Could you check a few things on this model? Use its own coordinates, in mm. Face numbers are marked on the shaded views. Give positions to 0.01 mm unless a question says otherwise; leave off trailing zeros. Loops run counter-clockwise (first coordinate to the right, second up) from the corner with the lowest first, then second, coordinate; pieces in that order, holes last.
1. Imagine slicing it at A-A (z = 0). List the corners of the cut face in (x, y) for me, plus the area to 4 significant figures.
2. Imagine slicing it at B-B (y = 1.5). List the corners of the cut face in (x, z) for me.
3. For P1, Ø2, axis at x = -12.5, z = 0, coming from the +Y side; P2, Ø4, axis at y = 7, z = 10.5, coming from the -X side; P3, Ø5, axis at y = 2, z = -7, coming from the +X side; P4, Ø3, axis at x = 0, z = 12.5, coming from the -Y side, each with a flat end and sliding along its axis, tell me the tip position at first contact or that it passes through.
4. Thinking about a two-plate mould opening in Z: for the marked faces 1, 2 and 3, which applies, +Z half, -Z half, draft (parallel to the pull), parting line (faces both ways), or undercut?
5. Imagine slicing it at D-D (z = -12.5). List the corners of the cut face in (x, y) for me.
6. I need wall thicknesses on line 1 along X through (y, z) = (6.5, 0); line 2 along X through (y, z) = (3.75, 1); line 3 along X through (y, z) = (7.25, -12.5). Which ranges of each line are inside material? Lowest first, please.
7. Imagine slicing it at C-C (x = 12.5). List the corners of the cut face in (y, z) for me.
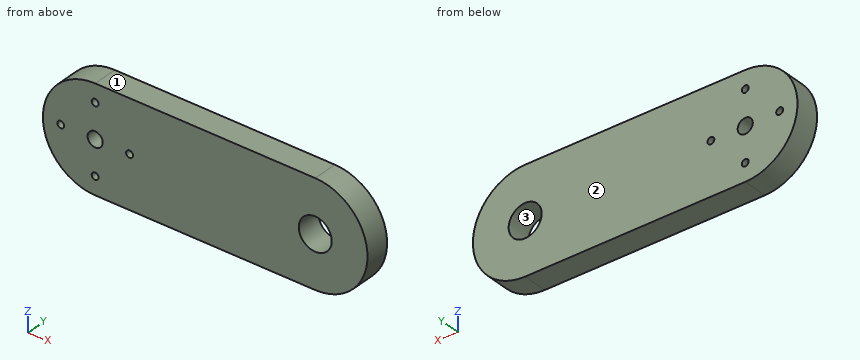
```python
from build123d import *

# Parameters (mm, degrees)
SKETCH_1_R         = 2.75
SKETCH_1_R_2       = 6
EXTRUDE_1_DEPTH    = 9
HOLE_WIZARD_M3_1_D = 2.5


with BuildPart() as part:
    # 草图1 → 凸台-拉伸1 (new body)
    with BuildSketch(Plane(origin=(0, 0, 0), x_dir=(1, 0, 0), z_dir=(0, 1, 0))):
        with BuildLine():
            Line((0, 19), (80, 19))
            ThreePointArc((80, 19), (99, 0), (80, -19))
            Line((80, -19), (0, -19))
            ThreePointArc((0, -19), (-19, 0), (0, 19))
        make_face()
        with Locations(Location((0, 0, 0), (0, 0, 270))):
            Circle(SKETCH_1_R, mode=Mode.SUBTRACT)
        with Locations(Location((80, 0, 0), (0, 0, 270))):
            Circle(SKETCH_1_R_2, mode=Mode.SUBTRACT)
    extrude(amount=EXTRUDE_1_DEPTH)

    # M3 螺纹孔的螺纹孔钻头1 (through all)
    with Locations(Plane(origin=(0, 9, -12.5), x_dir=(0, 0, 1), z_dir=(0, 1, 0))):
        with Locations((0, 0), (12.5, 12.5), (25, 0), (12.5, -12.5)):
            Hole(HOLE_WIZARD_M3_1_D / 2)


solid = part.part
```
Derived:
1. outline: (-19, 0) - (-13.75, 0) - (-13.75, 9) - (-19, 9) - close; (-11.25, 0) - (-2.75, 0) - (-2.75, 9) - (-11.25, 9) - close; (2.75, 0) - (11.25, 0) - (11.25, 9) - (2.75, 9) - close; (13.75, 0) - (74, 0) - (74, 9) - (13.75, 9) - close; (86, 0) - (99, 0) - (99, 9) - (86, 9) - close
1. area: 859.5 mm2
2. outline: (0, -19) - (80, -19) arc R19 ccw to (80, 19) - (0, 19) arc R19 ccw to start; hole circle Ø2.5 at (-12.5, 0); hole circle Ø5.5 at (0, 0); hole circle Ø2.5 at (0, -12.5); hole circle Ø2.5 at (0, 12.5); hole circle Ø2.5 at (12.5, 0); hole circle Ø12 at (80, 0)
3. P1: passes through
3. P2: stops at x = -16.99
3. P3: stops at x = 98.46
3. P4: stops at y = 0
4. face 1: +Z half
4. face 2: draft
4. face 3: undercut
5. outline: (-14.31, 0) - (-1.25, 0) - (-1.25, 9) - (-14.31, 9) - close; (1.25, 0) - (94.31, 0) - (94.31, 9) - (1.25, 9) - close
6. line 1: x = -19 to -13.75, -11.25 to -2.75, 2.75 to 11.25, 13.75 to 74, 86 to 99
6. line 2: x = -18.97 to -13.25, -11.75 to -2.56, 2.56 to 11.75, 13.25 to 74.08, 85.92 to 98.97
6. line 3: x = -14.31 to -1.25, 1.25 to 94.31
7. outline: (0, -19) - (9, -19) - (9, -1.25) - (0, -1.25) - close; (0, 1.25) - (9, 1.25) - (9, 19) - (0, 19) - close
